Check sheet for the modelled part. Datum: model origin and axes. Units: mm. A direction names the side the tool comes from. Give positions to 0.01 mm unless a question says otherwise; leave off trailing zeros. Write each loop counter-clockwise with the first axis right and the second up, starting at its lowest first coordinate (ties: lowest second). Pieces come first, ordered by that corner, then holes. Notation, with made-up numbers: M -37.75,16 L 21.25,16 A16 cw 21.25,33 Z; hole C 84,89.25 d3. An arc over 180 degrees is marked long. Write item = value, one per line. Start each with the question number.
1) Scan lines: line 1 along Y through (x, z) = (145, 3.2); line 2 along Y through (x, z) = (14, 1.15); line 3 along X through (y, z) = (-8, 1.25). Record each from-to range of solid material in increasing order. Write a range as [from, to].
2) Access from +Z, -Z, +X, -X, +Y, -Y to the whole of each face (thin tool, end or side, straight path). Record for faces 5 (the flat face through (13, -102, 3)), 6 (the flat face through (-2, -10, 3)), 7 (the flat face through (120.95, -3, 3)).
3) Cross-section at C-C, the plane y = -76. Record the cut outline in (x, z).
4) Cross-section at B-B, the plane z = 3.45. Give the number of separate pieces and of enclosed holes in the cut face, plus the area to 3 significant figures.
5) Mould release check, pull along Y, two halves, no side actions. Record for faces 1 (the flat face through (3, -28, 3)), 2 (the cylindrical face through (146.669, -14.474, 2.535)), 3 (the flat face through (76, -130, 2)), 4 (the cylindrical face through (149, -2, 3)): released by +Y, released by -Y, zero draft, split by the parting line, or undercut.
6) Cross-section at A-A, the plane y = -115. Record the cut outline in (x, z).
7) Go/stop test with flat-tipped pins: pin 1 (2.5 mm diameter, centred on x = 2.5, z = 3.5, fed in from -Y); pin 2 (2 mm diameter, centred on y = -101.5, z = 0.5, fed in from -X); pin 3 (1.5 mm diameter, centred on x = -2, z = 2, fed in from -Y). Record where each tip stops, or that it passes through.
Autodesk Inventor part; units mm, degrees
ref_plane "YZ Plane" through (0, 0, 0) normal (1, 0, 0) x (0, 1, 0)
ref_plane "XZ Plane" through (0, 0, 0) normal (0, 1, 0) x (-1, 0, 0)
ref_plane "XY Plane" through (0, 0, 0) normal (0, 0, 1) x (1, 0, 0)
sketch "Boceto1" plane through (0, 0, 0) normal (0, 0, 1) x (1, 0, 0)
  line L0 (0, 0) -> (150, 0)
  line L1 (150, 0) -> (150, -130)
  line L2 (150, -130) -> (0, -130)
  line L3 (0, -130) -> (0, 0)
  dimension "d2" = 130
  dimension "d3" = 150
extrude "Extrusión1" add sketch "Boceto1" along normal blind 5
fillet "Empalme1" radius 5 4 edges at (150, -130, 2.5) (150, 0, 2.5) (0, 0, 2.5) (0, -130, 2.5)
sketch "Boceto2" plane through (0, 0, 5) normal (0, 0, 1) x (1, 0, 0)
  line L0 (0, -125) -> (0, -5)
  line L1 (0, -10) -> (-5, -10)
  line L2 (-5, -10) -> (-5, -20)
  line L3 (-5, -20) -> (0, -20)
  line L4 (0, -20) -> (0, -10)
  line L5 (0, -110) -> (-5, -110)
  line L6 (-5, -110) -> (-5, -120)
  line L7 (-5, -120) -> (0, -120)
  line L8 (0, -120) -> (0, -110)
  line L9 (5, 0) -> (145, 0)
  point P0 (0, 0)
  dimension "d5" = 10
  dimension "d6" = 10
  dimension "d7" = 5
  dimension "d8" = 5
  dimension "d11" = 10
  dimension "d12" = 110
extrude "Extrusión2" add sketch "Boceto2" against normal blind 5
sketch "Boceto3" plane through (0, 0, 5) normal (0, 0, 1) x (1, 0, 0)
  line L0 (-5, -20) -> (0, -20)
  line L1 (0, -110) -> (0, -20)
  line L2 (-0.1512, -97.9504) -> (7.0488, -97.9504)
  line L3 (7.0488, -97.9504) -> (7.0488, -96.7034)
  line L4 (7.0488, -96.7034) -> (10.0488, -96.7034)
  line L5 (10.0488, -96.7034) -> (10.0488, -97.9504)
  line L6 (10.0488, -97.9504) -> (15.7176, -97.9504)
  line L7 (15.7176, -97.9504) -> (15.7176, -102)
  line L8 (15.7176, -102) -> (10.0488, -102)
  line L9 (10.0488, -102) -> (10.0488, -103.247)
  line L10 (10.0488, -103.247) -> (7.0488, -103.247)
  line L11 (7.0488, -103.247) -> (7.0488, -102)
  line L12 (7.0488, -102) -> (-0.1512, -102)
  line L13 (10.0793, -33.2966) -> (7.0793, -33.2966)
  line L14 (7.0793, -33.2966) -> (7.0793, -32.0496)
  line L15 (10.0793, -32.0496) -> (10.0793, -33.2966)
  line L16 (7.0793, -32.0496) -> (-0.1207, -32.0496)
  line L17 (15.7481, -32.0496) -> (10.0793, -32.0496)
  line L18 (-0.1207, -28) -> (7.0793, -28)
  line L19 (15.7481, -28) -> (15.7481, -32.0496)
  line L20 (7.0793, -28) -> (7.0793, -26.753)
  line L21 (7.0793, -26.753) -> (10.0793, -26.753)
  line L22 (10.0793, -26.753) -> (10.0793, -28)
  line L23 (10.0793, -28) -> (15.7481, -28)
  line L24 (-0.1207, -28) -> (-0.1207, -32.0496)
  line L25 (-0.1512, -97.9504) -> (-0.1512, -102)
  point P0 (0, 0)
  dimension "d15" = 8
  dimension "d16" = 8
extrude "Extrusión3" cut sketch "Boceto3" against normal blind 10
sketch "Boceto4" plane through (0, 0, 5) normal (0, 0, 1) x (1, 0, 0)
  line L0 (125, 0.788) -> (125, -6.2913)
  line L1 (125, -6.2913) -> (126.247, -6.2913)
  line L2 (126.247, -6.2913) -> (126.247, -9.2913)
  line L3 (126.247, -9.2913) -> (125, -9.2913)
  line L4 (125, -9.2913) -> (125, -14.9601)
  line L5 (125, -14.9601) -> (120.9504, -14.9601)
  line L6 (120.9504, -14.9601) -> (120.9504, -9.2913)
  line L7 (120.9504, -9.2913) -> (119.7034, -9.2913)
  line L8 (119.7034, -9.2913) -> (119.7034, -6.2913)
  line L9 (119.7034, -6.2913) -> (120.9504, -6.2913)
  line L10 (120.9504, -6.2913) -> (120.9504, 0.788)
  line L11 (120.9504, 0.788) -> (125, 0.788)
  point P0 (0, 0)
  point P1 (150, -5)
  dimension "d22" = 25
extrude "Extrusión4" cut sketch "Boceto4" against normal blind 10
sketch "Boceto5" plane through (0, 0, 5) normal (0, 0, 1) x (1, 0, 0)
  circle A0 centre (145, -115) radius 1.75
  circle A1 centre (145, -15) radius 1.75
  point P0 (0, 0)
  dimension "d24" = 3.5
  dimension "d25" = 3.5
extrude "Extrusión5" cut sketch "Boceto5" against normal blind 10
properties part number "pieza protectora ramps"
Reply:
q1.line_1 = [-130, -116.75], [-113.25, -16.75], [-13.25, 0]
q1.line_2 = [-130, -102], [-97.95, -32.05], [-28, 0]
q1.line_3 = [0, 119.7], [126.25, 150]
q2.face_5 = +Z, -Z, -X
q2.face_6 = +Z, -Z, -X, +Y
q2.face_7 = +Z, -Z, +Y
q3.outline = M 0,0 L 150,0 L 150,5 L 0,5 Z
q4.separate_pieces = 1
q4.enclosed_holes = 2
q4.area = 19,300 mm2
q5.face_1 = undercut
q5.face_2 = undercut
q5.face_3 = released by -Y
q5.face_4 = released by +Y
q6.outline = M -5,0 L 143.25,0 L 143.25,5 L -5,5 Z; M 146.75,0 L 150,0 L 150,5 L 146.75,5 Z
q7.pin_1 = -129.84
q7.pin_2 = 0
q7.pin_3 = -120
